Here's how the part is built. I have some questions about the finished solid (model axes, mm). Coordinates: 2 decimals unless noted, no trailing zeros. Write each loop counter-clockwise with the first axis right and the second up, starting at its lowest first coordinate (ties: lowest second). Pieces come first, ordered by that corner, then holes.
from build123d import *

# Parameters (mm, degrees)
SKETCH2_W                                       = 56
SKETCH2_H                                       = 22
BOSS_EXTRUDE2_DEPTH                             = 5
SKETCH5_R                                       = 2
MOUNTING_HOLES_DEPTH                            = 61.373835392
SMALL_EDGE_FILLET_R                             = 1
FRONT_BACK_EDGE_FILLET_R                        = 1
CSK_FOR_M4_FLAT_HEAD_MACHINE_SCREW2_D           = 4.5
CSK_FOR_M4_FLAT_HEAD_MACHINE_SCREW2_CSINK_D     = 9.4
CSK_FOR_M4_FLAT_HEAD_MACHINE_SCREW2_CSINK_ANGLE = 90


with BuildPart() as part:
    # Sketch2 → Boss-Extrude2 (new body)
    with BuildSketch(Plane.XY):
        with Locations((28, 11)):
            Rectangle(SKETCH2_W, SKETCH2_H)
    extrude(amount=-BOSS_EXTRUDE2_DEPTH)

    # Sketch5 → Mounting Holes (cut, through all)
    with BuildSketch(Plane.XY):
        with Locations((16.5, 11)):
            Circle(SKETCH5_R)
        with Locations((39.5, 11)):
            Circle(SKETCH5_R)
    extrude(amount=-MOUNTING_HOLES_DEPTH, mode=Mode.SUBTRACT)

    # Small Edge Fillet
    small_edge_fillet_edges = [part.edges().sort_by_distance(p)[0] for p in [
        (0, 22, -2.5),
        (56, 22, -2.5),
        (56, 0, -2.5),
        (0, 0, -2.5),
    ]]
    fillet(small_edge_fillet_edges, radius=SMALL_EDGE_FILLET_R)

    # Front-Back Edge Fillet
    front_back_edge_fillet_edges = [part.edges().sort_by_distance(p)[0] for p in [
        (0, 11, 0),
        (0, 11, -5),
        (28, 0, 0),
        (56, 11, 0),
        (28, 22, 0),
        (0.292893219, 21.707106781, 0),
        (55.707106781, 21.707106781, 0),
        (55.707106781, 0.292893219, 0),
        (0.292893219, 0.292893219, 0),
        (28, 0, -5),
        (28, 22, -5),
        (56, 11, -5),
        (0.292893219, 21.707106781, -5),
        (55.707106781, 21.707106781, -5),
        (55.707106781, 0.292893219, -5),
        (0.292893219, 0.292893219, -5),
    ]]
    fillet(front_back_edge_fillet_edges, radius=FRONT_BACK_EDGE_FILLET_R)

    # CSK for M4 Flat Head Machine Screw2 (through all)
    with Locations(Plane(origin=(0, 0, -5), x_dir=(-1, 0, 0), z_dir=(0, 0, -1))):
        with Locations((-28, 11)):
            CounterSinkHole(CSK_FOR_M4_FLAT_HEAD_MACHINE_SCREW2_D / 2, CSK_FOR_M4_FLAT_HEAD_MACHINE_SCREW2_CSINK_D / 2, counter_sink_angle=CSK_FOR_M4_FLAT_HEAD_MACHINE_SCREW2_CSINK_ANGLE)


solid = part.part
1. I want a section at A-A (x = 16.5). List the corners of the cut face in (y, z) for me.
2. Thinking about a two-plate mould opening in Y: for faces 1 (the face through (28, 22, -2)), 2 (the face through (25.6, 11.1, -2.7)), 3 (the face through (34, 11, -5)), which applies, pulls with the +Y half, pulls with the -Y half, needs draft (parallel to the pull), parting line crosses it, or undercut?
3. I want a section at D-D (z = -0.5). List the corners of the cut face in (x, y) for me, then the cut area to 3 significant figures.
4. I want a section at B-B (y = 11). List the corners of the cut face in (x, z) for me.
5. For pin 1 Ø4.5 at (x, y) = (16.5, 11) entering from +Z; pin 2 Ø6 at (x, y) = (28, 11) entering from -Z, each with a flat end and sliding along its axis, tell me the tip position at first contact or that it passes through.
6. I want a section at C-C (z = -3.4). List the corners of the cut face in (x, y) for me.
7. If I drill on line 1 (Y direction, x = 16.5, z = -1.45); line 2 (X direction, y = 11.5, z = -0.7); line 3 (Y direction, x = 28, z = -0.55), over which ranges is the centre line in solid material (lowest first)?
Response values:
1. outline: (0, -4) arc R1 ccw to (1, -5) - (9, -5) - (9, 0) - (1, 0) arc R1 ccw to (0, -1) - close; (13, -5) - (21, -5) arc R1 ccw to (22, -4) - (22, -1) arc R1 ccw to (21, 0) - (13, 0) - close
2. face 1: pulls with the +Y half
2. face 2: undercut
2. face 3: needs draft
3. outline: (0.13, 1) arc R0.87 ccw to (1, 0.13) - (55, 0.13) arc R0.87 ccw to (55.87, 1) - (55.87, 21) arc R0.87 ccw to (55, 21.87) - (1, 21.87) arc R0.87 ccw to (0.13, 21) - close; hole circle Ø4 at (16.5, 11); hole circle Ø4.5 at (28, 11); hole circle Ø4 at (39.5, 11)
3. area: 1,170 mm2
4. outline: (0, -4) arc R1 ccw to (1, -5) - (14.5, -5) - (14.5, 0) - (1, 0) arc R1 ccw to (0, -1) - close; (18.5, -5) - (23.3, -5) - (25.75, -2.55) - (25.75, 0) - (18.5, 0) - close; (30.25, -2.55) - (32.7, -5) - (37.5, -5) - (37.5, 0) - (30.25, 0) - close; (41.5, -5) - (55, -5) arc R1 ccw to (56, -4) - (56, -1) arc R1 ccw to (55, 0) - (41.5, 0) - close
5. pin 1: stops at z = 0
5. pin 2: stops at z = -3.3
6. outline: (0, 1) arc R1 ccw to (1, 0) - (55, 0) arc R1 ccw to (56, 1) - (56, 21) arc R1 ccw to (55, 22) - (1, 22) arc R1 ccw to (0, 21) - close; hole circle Ø4 at (16.5, 11); hole circle Ø6.2 at (28, 11); hole circle Ø4 at (39.5, 11)
7. line 1: y = 0 to 9, 13 to 22
7. line 2: x = 0.05 to 14.56, 18.44 to 25.81, 30.19 to 37.56, 41.44 to 55.95
7. line 3: y = 0.11 to 8.75, 13.25 to 21.89
